Check sheet for the modelled part. Datum: model origin and axes. Units: mm. A direction names the side the tool comes from. Round coordinates to 2 decimals unless told otherwise and drop trailing zeros. Order: outer loops, then holes, each group sorted by start corner. A loop starts at its lowest first (then second) coordinate and runs counter-clockwise, first axis right, second up. Notation, with made-up numbers: (6, 66.25) -> (42, 66.25) arc R25 cw to (42, 78.25) -> close; hole circle Ø7 at (-7, 88.25). An arc over 180 degrees is marked (long way). Answer in a Markdown table with one row per item.
Solid Edge part; units mm, degrees
sketch "Sketch1" plane through (0, 0, 0) normal (0, 0, 1) x (1, 0, 0)
  line L0 (-6.1009, 4.0673) -> (-6.5728, -3.2499)
  line L1 (-6.5728, -3.2499) -> (-0.4719, -7.3171)
  line L2 (-0.4719, -7.3171) -> (6.1009, -4.0673)
  line L3 (6.1009, -4.0673) -> (6.5728, 3.2499)
  line L4 (6.5728, 3.2499) -> (0.4719, 7.3171)
  line L5 (0.4719, 7.3171) -> (-6.1009, 4.0673)
extrude "Protrusion1" add sketch "Sketch1" against normal blind 390
sketch "Sketch2" plane through (0, 0, -2) normal (0, 0, 1) x (-0.8964, -0.4432, 0)
  circle A0 centre (0, 0) radius 5.5
  circle A1 centre (0, 0) radius 13.1424
extrude "ExtrudedCutout_1" cut sketch "Sketch2" against normal blind 2
sketch "Sketch3" plane through (0, 0, -388) normal (0, 0, -1) x (0.8964, 0.4432, 0)
  circle A0 centre (0, 0) radius 5.5
  circle A1 centre (0, 0) radius 13.1424
extrude "ExtrudedCutout_2" cut sketch "Sketch3" against normal blind 2
properties part number "BumbleB0247"
Item 1: Depth check by flat-ended pin: P1, Ø5, axis at x = 4.5, y = 5, coming from the -Z side; P2, Ø2, axis at y = 0.5, z = -314, coming from the -X side; P3, Ø4, axis at y = -3.5, z = -274.5, coming from the +X side; P4, Ø1, axis at x = -2.5, z = -45.5, coming from the +Y side. Enter the tip coordinate at first touch or a pass-through.
Result sheet:
| item | result |
|---|---|
| P1 | stops at z = -390 |
| P2 | stops at x = -6.4 |
| P3 | stops at x = 6.27 |
| P4 | stops at y = 6.09 |
Item 2: Cross-section at A-A (z = -340.5). Record the boundary of the cut face in (x, y), and give its area (3 significant figures).
Result sheet:
| item | result |
|---|---|
| outline | (-6.57, -3.25) -> (-0.47, -7.32) -> (6.1, -4.07) -> (6.57, 3.25) -> (0.47, 7.32) -> (-6.1, 4.07) -> close |
| area | 140 mm^2 |
Item 3: Cross-section at B-B (y = 0). Record the boundary of the cut face in (x, z).
Result sheet:
| item | result |
|---|---|
| outline | (-6.36, -390) -> (6.36, -390) -> (6.36, -388) -> (5.5, -388) -> (5.5, -386) -> (6.36, -386) -> (6.36, -4) -> (5.5, -4) -> (5.5, -2) -> (6.36, -2) -> (6.36, 0) -> (-6.36, 0) -> (-6.36, -2) -> (-5.5, -2) -> (-5.5, -4) -> (-6.36, -4) -> (-6.36, -386) -> (-5.5, -386) -> (-5.5, -388) -> (-6.36, -388) -> close |
Item 4: Set-up check for faces 1 (the flat face through (-5, -3, -2)), 2 (the flat face through (0, 0, 0)): record each of +Z, -Z, +X, -X, +Y, -Y from which the full face is reachable in a straight line by a thin tool's end or side.
Result sheet:
| item | result |
|---|---|
| face 1 | none |
| face 2 | +Z, +X, -X, +Y, -Y |
Item 5: Mould release check, pull along Z, two halves, no side actions. Record for faces 3 (the flat face through (0, 0, -390)), 4 (the flat face through (-3.565, -5.255, -192.326)), 5 (the flat face through (5, -3, -388)): pulls with the +Z half, pulls with the -Z half, needs draft (parallel to the pull), parting line crosses it, or undercut.
Result sheet:
| item | result |
|---|---|
| face 3 | pulls with the -Z half |
| face 4 | needs draft |
| face 5 | undercut |
Item 6: Scan lines: line 1 (Z direction, x = -3, y = 5); line 2 (X direction, y = -3.25, z = -105.5); line 3 (Y direction, x = -3.25, z = -192). Record each from-to range of solid material in increasing order. Write a range as [from, to].
Result sheet:
| item | result |
|---|---|
| line 1 | z = [-390, -388], [-386, -4], [-2, 0] |
| line 2 | x = [-6.57, 6.15] |
| line 3 | y = [-5.47, 5.48] |
